Part model, mm, in its own coordinate system. A direction names the side the tool comes from. Coordinates: 2 decimals unless noted, no trailing zeros. Write each loop counter-clockwise with the first axis right and the second up, starting at its lowest first coordinate (ties: lowest second). Pieces come first, ordered by that corner, then holes. Notation, with made-up numbers: (-15.5, 10.5) - (19.5, 10.5) arc R22 cw to (19.5, 24.5) - close; hole circle Ø5 at (56, -14). An arc over 180 degrees is marked (long way). Write each question's results on one line, items separated by ' | '.
from build123d import *

# Parameters (mm, degrees)
ESBO_O1_W                  = 51
ESBO_O1_H                  = 51
RESSALTO_EXTRUS_O1_DEPTH   = 8
ESBO_O2_W                  = 4
ESBO_O2_H                  = 20
RESSALTO_EXTRUS_O2_DEPTH   = 80
ESBO_O4_W                  = 20
ESBO_O4_H                  = 4
RESSALTO_EXTRUS_O3_DEPTH   = 15
ESBO_O5_R                  = 1.6
CORTE_EXTRUS_O2_DEPTH      = 7
FILETE2_R                  = 10
CORTE_EXTRUS_O3_DEPTH      = 105.858237635
CORTE_EXTRUS_O3_DEPTH_BACK = 105.858237635
ESBO_O6_W                  = 13
ESBO_O6_H                  = 30
ESBO_O7_R                  = 1.5
CORTE_EXTRUS_O4_DEPTH      = 105.858237635
FILETE6_R                  = 10


with BuildPart() as part:
    # Esboço1 → Ressalto-extrusão1 (new body)
    with BuildSketch(Plane(origin=(0, 0, 0), x_dir=(1, 0, 0), z_dir=(0, 1, 0))):
        Rectangle(ESBO_O1_W, ESBO_O1_H)
    extrude(amount=RESSALTO_EXTRUS_O1_DEPTH)

    # Esboço2 → Ressalto-extrusão2 (add)
    with BuildSketch(Plane(origin=(0, 8, 0), x_dir=(1, 0, 0), z_dir=(0, 1, 0))):
        with Locations((-23.5, 0)):
            Rectangle(ESBO_O2_W, ESBO_O2_H)
        with Locations((23.5, 0)):
            Rectangle(ESBO_O2_W, ESBO_O2_H)
    extrude(amount=RESSALTO_EXTRUS_O2_DEPTH)

    # Esboço4 → Ressalto-extrusão3 (add)
    with BuildSketch(Plane(origin=(0, 8, 0), x_dir=(1, 0, 0), z_dir=(0, 1, 0))):
        with Locations((0, 23.5)):
            Rectangle(ESBO_O4_W, ESBO_O4_H)
        with Locations((0, -23.5)):
            Rectangle(ESBO_O4_W, ESBO_O4_H)
    extrude(amount=RESSALTO_EXTRUS_O3_DEPTH)

    # Esboço5 → Corte-extrusão2 (cut)
    with BuildSketch(Plane.XZ):
        with Locations(Location((-11, 11, 0), (0, 0, 270))):
            Circle(ESBO_O5_R)
        with Locations(Location((11, 11, 0), (0, 0, 90))):
            Circle(ESBO_O5_R)
        with Locations(Location((11, -11, 0), (0, 0, 270))):
            Circle(ESBO_O5_R)
        with Locations(Location((-11, -11, 0), (0, 0, 90))):
            Circle(ESBO_O5_R)
    extrude(amount=-CORTE_EXTRUS_O2_DEPTH, mode=Mode.SUBTRACT)

    # Filete2
    filete2_edges = [part.edges().sort_by_distance(p)[0] for p in [
        (25.5, 4, 25.5),
        (-25.5, 4, 25.5),
        (-25.5, 4, -25.5),
        (25.5, 4, -25.5),
    ]]
    fillet(filete2_edges, radius=FILETE2_R)

    # Esboço6 → Corte-extrusão3 (cut, two sides: drawn at the far end of the back side and taken through both)
    with BuildSketch(Plane.ZY.offset(25.5).offset(-CORTE_EXTRUS_O3_DEPTH_BACK)):
        with Locations((0, 28)):
            Rectangle(ESBO_O6_W, ESBO_O6_H)
    extrude(amount=CORTE_EXTRUS_O3_DEPTH + CORTE_EXTRUS_O3_DEPTH_BACK, mode=Mode.SUBTRACT)

    # Esboço7 → Corte-extrusão4 (cut, through all)
    with BuildSketch(Plane(origin=(25.5, 0, 0), x_dir=(0, 0, -1), z_dir=(1, 0, 0))):
        with Locations((0, 78)):
            Circle(ESBO_O7_R)
    extrude(amount=-CORTE_EXTRUS_O4_DEPTH, mode=Mode.SUBTRACT)

    # Filete6
    filete6_edges = [part.edges().sort_by_distance(p)[0] for p in [
        (23.5, 88, -10),
        (23.5, 88, 10),
        (-23.5, 88, -10),
        (-23.5, 88, 10),
    ]]
    fillet(filete6_edges, radius=FILETE6_R - 0.0001)  # a hair under: the kernel refuses the full size


solid = part.part
(1) Wall check: line 1 (Y direction, x = 23, z = 0); line 2 (X direction, y = 5.25, z = 11); line 3 (X direction, y = 67, z = -4). Give the ranges that are in metal, low to high. Write a range as from..to.
Return value:
line 1: y = 0..13, 43..76.5, 79.5..88 | line 2: x = -25.5..-12.6, -9.4..9.4, 12.6..25.5 | line 3: x = -25.5..-21.5, 21.5..25.5
(2) Saw through at D-D on z = -11. Write the cut outline in (x, y).
Return value:
outline: (-25.5, 0) - (-12.6, 0) - (-12.6, 7) - (-9.4, 7) - (-9.4, 0) - (9.4, 0) - (9.4, 7) - (12.6, 7) - (12.6, 0) - (25.5, 0) - (25.5, 8) - (-25.5, 8) - close
(3) Saw through at C-C on x = -8. Write the cut outline in (y, z).
Return value:
outline: (0, -25.5) - (23, -25.5) - (23, -21.5) - (8, -21.5) - (8, 21.5) - (23, 21.5) - (23, 25.5) - (0, 25.5) - close
(4) Saw through at B-B on y = 31. Write the cut outline in (x, z), then the cut area to 3 significant figures.
Return value:
outline: (-25.5, -10) - (-21.5, -10) - (-21.5, -6.5) - (-25.5, -6.5) - close; (-25.5, 6.5) - (-21.5, 6.5) - (-21.5, 10) - (-25.5, 10) - close; (21.5, -10) - (25.5, -10) - (25.5, -6.5) - (21.5, -6.5) - close; (21.5, 6.5) - (25.5, 6.5) - (25.5, 10) - (21.5, 10) - close | area: 56.0 mm^2
(5) Saw through at A-A on y = 44.5. Write the cut outline in (x, z), then the cut area to 3 significant figures.
Return value:
outline: (-25.5, -10) - (-21.5, -10) - (-21.5, 10) - (-25.5, 10) - close; (21.5, -10) - (25.5, -10) - (25.5, 10) - (21.5, 10) - close | area: 160 mm^2
(6) 3-axis set-ups, long thin cutter, end or side, ignore diameter. For faces 1 (the flat face through (-23, 28, 6.5)), 2 (the cylindrical face through (11.97, 3.45, 9.73)), 3 (the flat face through (0, 15, 21.5)): which of +Z, -Z, +X, -X, +Y, -Y reach the whole face in a straight line?
Return value:
face 1: +X, -X | face 2: -Y | face 3: +X, -X, +Y
(7) Flat gauge pins, fed straight in: P1, Ø5, axis at y = 23.5, z = -11.5, coming from the +X side; P2, Ø4.5, axis at y = 19, z = 23.5, coming from the -X side; P3, Ø2, axis at x = -24, y = 29.5, coming from the +Z side; P4, Ø3, axis at x = -1.5, z = 23, coming from the +Y side. Where does each tip first touch, or does it go through?
Return value:
P1: stops at x = 25.5 | P2: stops at x = -10 | P3: stops at z = 10 | P4: stops at y = 23
(8) Two-plate mould, pull along Y, no slides. Class faces 4 (the flat face through (-11, 7, 11)), 5 (the cylindrical face through (-22.65, 4.06, 22.49)), 6 (the flat face through (24, 28, -6.5)): released by +Y, released by -Y, zero draft, split by the parting line, or undercut.
Return value:
face 4: released by -Y | face 5: zero draft | face 6: undercut
